Autodesk Inventor part; units mm, degrees
ref_plane "YZ Plane" through (0, 0, 0) normal (1, 0, 0) x (0, 1, 0)
ref_plane "XZ Plane" through (0, 0, 0) normal (0, 1, 0) x (-1, 0, 0)
ref_plane "XY Plane" through (0, 0, 0) normal (0, 0, 1) x (1, 0, 0)
sketch "Эскиз1" plane through (0, 0, 0) normal (1, 0, 0) x (0, 1, 0)
  line L0 (-17.5, 21) -> (-21, 17.5)
  line L1 (-21, 17.5) -> (-21, -17.5)
  line L2 (-21, -17.5) -> (-17.5, -21)
  line L3 (-17.5, -21) -> (17.5, -21)
  line L4 (17.5, -21) -> (21, -17.5)
  line L5 (21, -17.5) -> (21, 17.5)
  line L6 (21, 17.5) -> (17.5, 21)
  line L7 (17.5, 21) -> (-17.5, 21)
  circle A0 centre (0, 0) radius 11.3
  circle A1 centre (-15.5, -15.5) radius 1.25
  circle A2 centre (15.5, -15.5) radius 1.25
  circle A3 centre (15.5, 15.5) radius 1.25
  circle A4 centre (-15.5, 15.5) radius 1.25
  line L8 (-21, 17.5) -> (-51, 17.5)
  line L9 (-51, 17.5) -> (-51, -17.5)
  line L10 (-51, -17.5) -> (-21, -17.5)
  line L11 (-21, -17.5) -> (-21, 17.5)
  line L12 (-51, 0) -> (-36, 0)
  line L13 (-36, 0) -> (-36, 10)
  line L14 (-36, 10) -> (-36, -10)
  circle A5 centre (-36, 10) radius 3
  circle A6 centre (-36, -10) radius 3
  circle A7 centre (0, 0) radius 3
  dimension "d0" = 30
  dimension "d1" = 15
  dimension "d2" = 10
  dimension "d3" = 20
  dimension "d4" = 6
  dimension "d5" = 6
  dimension "d6" = 6
extrude "Выдавливание1" add sketch "Эскиз1" along normal blind 4 contours L7 L6 L5 L4 L3 L2 L1 L0 | L1 L10 L9 L8 | A0
chamfer "Фаска1" distance 5 angle 45 2 edges at (2, -51, 17.5) (2, -51, -17.5)
properties part number "КВ33.044.002 - Держатель катка"
Verification items for the finished model (mm, model axes). A direction names the side the tool comes from. Coordinates: 2 decimals unless noted, no trailing zeros. Loops run counter-clockwise (first coordinate to the right, second up) from the corner with the lowest first, then second, coordinate; pieces in that order, holes last. Notation, with made-up numbers: (-39, 36) - (-25, 36) arc R21 ccw to (-25, 69) - close; hole circle Ø9 at (77, 2.25). An arc over 180 degrees is marked (long way). Return JSON: item names as keys, results as strings.
1. Section check C-C, the plane y = 15.5. Record the boundary of the cut face in (x, z).
Established:
{"outline": "(0, -21) - (4, -21) - (4, -16.75) - (0, -16.75) - close; (0, -14.25) - (4, -14.25) - (4, 14.25) - (0, 14.25) - close; (0, 16.75) - (4, 16.75) - (4, 21) - (0, 21) - close"}
2. Section check B-B, the plane z = 0. Record the boundary of the cut face in (x, y).
Established:
{"outline": "(0, -51) - (4, -51) - (4, -3) - (0, -3) - close; (0, 3) - (4, 3) - (4, 21) - (0, 21) - close"}
3. Section check A-A, the plane z = 15.5. Record the boundary of the cut face in (x, y).
Established:
{"outline": "(0, -48) - (4, -48) - (4, -16.75) - (0, -16.75) - close; (0, -14.25) - (4, -14.25) - (4, 14.25) - (0, 14.25) - close; (0, 16.75) - (4, 16.75) - (4, 21) - (0, 21) - close"}
4. Section check D-D, the plane x = 3. Record the boundary of the cut face in (y, z).
Established:
{"outline": "(-51, -12.5) - (-46, -17.5) - (-21, -17.5) - (-17.5, -21) - (17.5, -21) - (21, -17.5) - (21, 17.5) - (17.5, 21) - (-17.5, 21) - (-21, 17.5) - (-46, 17.5) - (-51, 12.5) - close; hole circle Ø6 at (-36, -10); hole circle Ø6 at (-36, 10); hole circle Ø2.5 at (-15.5, -15.5); hole circle Ø2.5 at (-15.5, 15.5); hole circle Ø6 at (0, 0); hole circle Ø2.5 at (15.5, -15.5); hole circle Ø2.5 at (15.5, 15.5)"}
5. Thickness scan on L1, parallel to Z at x = 3.1, y = -36; L2, parallel to Z at x = 2.7, y = 15.5; L3, parallel to Y at x = 1.8, z = 16.5. Record the ranges inside material, lowest first.
Established:
{"L1": "z = -17.5 to -13, -7 to 7, 13 to 17.5", "L2": "z = -21 to -16.75, -14.25 to 14.25, 16.75 to 21", "L3": "y = -47 to -16.25, -14.75 to 14.75, 16.25 to 21"}
6. Tool access check on faces 1 (the cylindrical face through (1.97, 15.34, 14.26)), 2 (the flat face through (2, -33, 17.5)), 3 (the flat face through (2, -34, -17.5)). Record the directions out of +Z, -Z, +X, -X, +Y, -Y that give a thin tool (end or side, any length) a straight path to the whole face; none if there is none.
Established:
{"face 1": "+X, -X", "face 2": "+Z, +X, -X, -Y", "face 3": "-Z, +X, -X, -Y"}
7. Mould release check, pull along Y, two halves, no side actions. Record for faces 4 (the cylindrical face through (2, -39, -10)), 5 (the flat face through (2, -19.3, -19.2)), 6 (the flat face through (2, 19.3, 19.2)): +Y half, -Y half, draft (parallel to the pull), parting line (faces both ways), or undercut.
Established:
{"face 4": "undercut", "face 5": "-Y half", "face 6": "+Y half"}
